The listing builds one solid part. Answer for the finished solid, in the listing's coordinates (mm). A direction names the side the tool comes from. Give positions to 0.01 mm unless a question says otherwise; leave off trailing zeros. Loops run counter-clockwise (first coordinate to the right, second up) from the corner with the lowest first, then second, coordinate; pieces in that order, holes last. Notation, with made-up numbers: M 75,74.25 L 115,74.25 A16 cw 115,92.25 Z; hole C -15,-22 d4. An arc over 180 degrees is marked long. Use one line per item in the form item = value. Start each with the question number.
1. The part is cut by section B-B (x = 0). Write down the section's boundary in (y, z).
2. For faces 5 (the face through (-0.518, 3.521, -3.946)), 6 (the face through (0.208, 2.535, 14.086)), determine the directions among +Z, -Z, +X, -X, +Y, -Y from which every point of the face is accessible in a straight line to the end or side of a thin tool.
3. The part is cut by section D-D (y = 4.5). Write down the section's boundary in (x, z), and give its area (3 significant figures).
4. The part is cut by section A-A (z = 0). Write down the section's boundary in (x, y), and give its area (3 significant figures).
5. Straight lines are drawn through the part: line 1 (X direction, y = 2.6, z = 0); line 2 (Z direction, x = 0, y = 0.4). For each, find the intervals that lie inside material, in ascending order. Write a range as from..to.
6. The part is cut by section C-C (x = -12.5). Write down the section's boundary in (y, z).
7. Each of these flat-tipped pins is pushed along its axis until it touches: pin 1 Ø2.5 at (x, z) = (0, 0) entering from +Y; pin 2 Ø2.5 at (x, z) = (-1, -0.5) entering from +Y; pin 3 Ø1.5 at (y, z) = (3.5, -8) entering from +X; pin 4 Ø1 at (x, y) = (0, 1) entering from +Z. Where does it stop, or does it pass through?
8. The mould has two halves that part along Z. Classify faces 1 (the face through (1, 2, -2)), 2 (the face through (-2.539, 2.465, -19.334)), 3 (the face through (4, 0, 0)), 4 (the face through (-0.208, 2.535, -14.086)): released by +Z, released by -Z, zero draft, split by the parting line, or undercut.
from build123d import *

# Parameters (mm, degrees)
SKETCH1_R           = 19.5
BOSS_EXTRUDE1_DEPTH = 5
SKETCH2_R           = 3.98
CUT_EXTRUDE1_DEPTH  = 3
SKETCH3_R           = 2
CUT_EXTRUDE2_DEPTH  = 3
SKETCH4_R           = 1.6
CUT_EXTRUDE3_DEPTH  = 6
CIRPATTERN1_COUNT   = 4


with BuildPart() as part:
    # Sketch1 → Boss-Extrude1 (new body)
    with BuildSketch(Plane(origin=(0, 0, 0), x_dir=(1, 0, 0), z_dir=(0, 1, 0))):
        Circle(SKETCH1_R)
    extrude(amount=BOSS_EXTRUDE1_DEPTH)

    # Sketch2 → Cut-Extrude1 (cut)
    with BuildSketch(Plane(origin=(0, 5, 0), x_dir=(1, 0, 0), z_dir=(0, 1, 0))):
        Circle(SKETCH2_R)
    extrude(amount=-CUT_EXTRUDE1_DEPTH, mode=Mode.SUBTRACT)

    # Sketch3 → Cut-Extrude2 (cut)
    with BuildSketch(Plane(origin=(0, 2, 0), x_dir=(1, 0, 0), z_dir=(0, 1, 0))):
        Circle(SKETCH3_R)
    extrude(amount=-CUT_EXTRUDE2_DEPTH, mode=Mode.SUBTRACT)

    # Sketch4 → Cut-Extrude3 (cut, through all)
    with BuildSketch(Plane(origin=(0, 5, 0), x_dir=(1, 0, 0), z_dir=(0, 1, 0))):
        with Locations((0, 12.5)):
            Circle(SKETCH4_R)
    cut_extrude3 = extrude(amount=-CUT_EXTRUDE3_DEPTH, mode=Mode.SUBTRACT)

    # CirPattern1: Cut-Extrude3 ×4 about axis
    cirpattern1_axis = Axis((0, 0, 0), (0, 1, 0))
    for i in range(1, CIRPATTERN1_COUNT):
        add(cut_extrude3.rotate(cirpattern1_axis, i * 360 / CIRPATTERN1_COUNT), mode=Mode.SUBTRACT)


solid = part.part
Derived:
q1.outline = M 0,-19.5 L 5,-19.5 L 5,-14.1 L 0,-14.1 Z; M 0,-10.9 L 5,-10.9 L 5,-3.98 L 2,-3.98 L 2,-2 L 0,-2 Z; M 0,2 L 2,2 L 2,3.98 L 5,3.98 L 5,10.9 L 0,10.9 Z; M 0,14.1 L 5,14.1 L 5,19.5 L 0,19.5 Z
q2.face_5 = +Y
q2.face_6 = +Y, -Y
q3.outline = C 0,0 d39; hole C -12.5,0 d3.2; hole C 0,0 d7.96; hole C 0,-12.5 d3.2; hole C 0,12.5 d3.2; hole C 12.5,0 d3.2
q3.area = 1,110 mm2
q4.outline = M -19.5,0 L -14.1,0 L -14.1,5 L -19.5,5 Z; M -10.9,0 L -2,0 L -2,2 L -3.98,2 L -3.98,5 L -10.9,5 Z; M 2,0 L 10.9,0 L 10.9,5 L 3.98,5 L 3.98,2 L 2,2 Z; M 14.1,0 L 19.5,0 L 19.5,5 L 14.1,5 Z
q4.area = 131 mm2
q5.line_1 = -19.5..-14.1, -10.9..-3.98, 3.98..10.9, 14.1..19.5
q5.line_2 = -19.5..-14.1, -10.9..-2, 2..10.9, 14.1..19.5
q6.outline = M 0,-14.97 L 5,-14.97 L 5,-1.6 L 0,-1.6 Z; M 0,1.6 L 5,1.6 L 5,14.97 L 0,14.97 Z
q7.pin_1 = through
q7.pin_2 = 2
q7.pin_3 = 18.1
q7.pin_4 = 19.5
q8.face_1 = undercut
q8.face_2 = split by the parting line
q8.face_3 = zero draft
q8.face_4 = undercut
